Part model, mm, in its own coordinate system. Face numbers are marked on the shaded views. Coordinates: 2 decimals unless noted, no trailing zeros. Loops run counter-clockwise (first coordinate to the right, second up) from the corner with the lowest first, then second, coordinate; pieces in that order, holes last. Notation, with made-up numbers: (6, 80) -> (56, 80) arc R24 cw to (56, 92) -> close; hole circle Ø4 at (4.5, -2.5). An arc over 180 degrees is marked (long way). One line per item, written item: value. Start each with the question number.
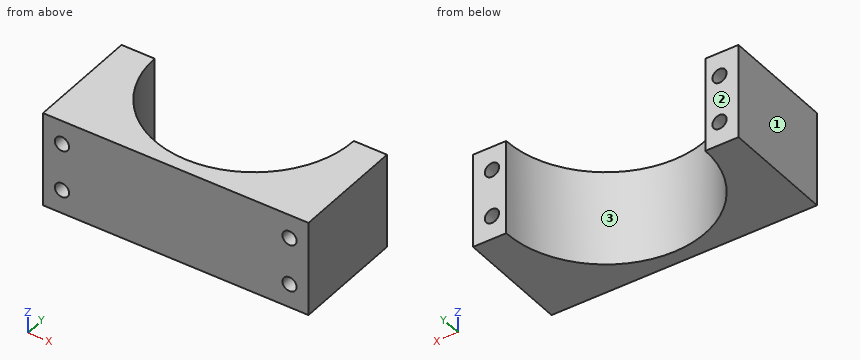
from build123d import *

# Parameters (mm, degrees)
EXTRUDE_1_DEPTH     = 20
SKETCH_2_R          = 1.5
CUT_EXTRUDE_1_DEPTH = 25


with BuildPart() as part:
    # 草图1 → 凸台-拉伸1 (new body)
    with BuildSketch(Plane.XY):
        with BuildLine():
            Line((-28, -24), (28, -24))
            Line((28, -24), (28, 0))
            Line((28, 0), (21, 0))
            ThreePointArc((21, 0), (0, -21), (-21, 0))
            Line((-21, 0), (-28, 0))
            Line((-28, 0), (-28, -24))
        make_face()
    extrude(amount=EXTRUDE_1_DEPTH)

    # 草图2 → 切除-拉伸1 (cut, through all)
    with BuildSketch(Plane(origin=(0, 0, 0), x_dir=(1, 0, 0), z_dir=(0, 1, 0))):
        with Locations((-24, -5)):
            Circle(SKETCH_2_R)
        with Locations((-24, -15)):
            Circle(SKETCH_2_R)
    cut_extrude_1 = extrude(amount=-CUT_EXTRUDE_1_DEPTH, mode=Mode.SUBTRACT)

    # 镜向1: 切除-拉伸1 across plane
    add(cut_extrude_1.mirror(Plane(origin=(0, 0, 0), x_dir=(0, 0, 1), z_dir=(1, 0, 0))), mode=Mode.SUBTRACT)


solid = part.part
1) Slice it at A-A (z = 15). Give the cut face in (x, y).
2) Slice it at C-C (x = 24). Give the cut face in (y, z).
3) Slice it at D-D (y = -21.75). Give the cut face in (x, z).
4) Slice it at B-B (y = -5.5). Give the cut face in (x, z).
5) Pin check, flat tips, straight feed: pin 1 Ø5 at (x, z) = (-0.5, 12.5) entering from +Y; pin 2 Ø2.5 at (x, z) = (24, 5) entering from +Y. Stop position of each tip, or through.
6) Probe line 1 (Z direction, x = -24, y = -14.25); line 2 (X direction, y = -13.75, z = 15); line 3 (X direction, y = -10.5, z = 14.5). List the from-to ranges inside material, lowest first. Write a range as from..to.
7) Pull direction X, two halves, no side cores. Call the marked faces 1, 2 and 3: +X half, -X half, draft (parallel to the pull), parting line (faces both ways), or undercut.
Check sheet entries:
1. outline: (-28, -24) -> (-25.5, -24) -> (-25.5, 0) -> (-28, 0) -> close; (-22.5, -24) -> (22.5, -24) -> (22.5, 0) -> (21, 0) arc R21 cw to (-21, 0) -> (-22.5, 0) -> close; (25.5, -24) -> (28, -24) -> (28, 0) -> (25.5, 0) -> close
2. outline: (-24, 0) -> (0, 0) -> (0, 3.5) -> (-24, 3.5) -> close; (-24, 6.5) -> (0, 6.5) -> (0, 13.5) -> (-24, 13.5) -> close; (-24, 16.5) -> (0, 16.5) -> (0, 20) -> (-24, 20) -> close
3. outline: (-28, 0) -> (28, 0) -> (28, 20) -> (-28, 20) -> close; hole circle Ø3 at (-24, 5); hole circle Ø3 at (-24, 15); hole circle Ø3 at (24, 5); hole circle Ø3 at (24, 15)
4. outline: (-28, 0) -> (-20.27, 0) -> (-20.27, 20) -> (-28, 20) -> close; (20.27, 0) -> (28, 0) -> (28, 20) -> (20.27, 20) -> close; hole circle Ø3 at (-24, 5); hole circle Ø3 at (-24, 15); hole circle Ø3 at (24, 5); hole circle Ø3 at (24, 15)
5. pin 1: stops at y = -20.78
5. pin 2: passes through
6. line 1: z = 0..3.5, 6.5..13.5, 16.5..20
6. line 2: x = -28..-25.5, -22.5..-15.87, 15.87..22.5, 25.5..28
6. line 3: x = -28..-25.41, -22.59..-18.19, 18.19..22.59, 25.41..28
7. face 1: -X half
7. face 2: draft
7. face 3: undercut
